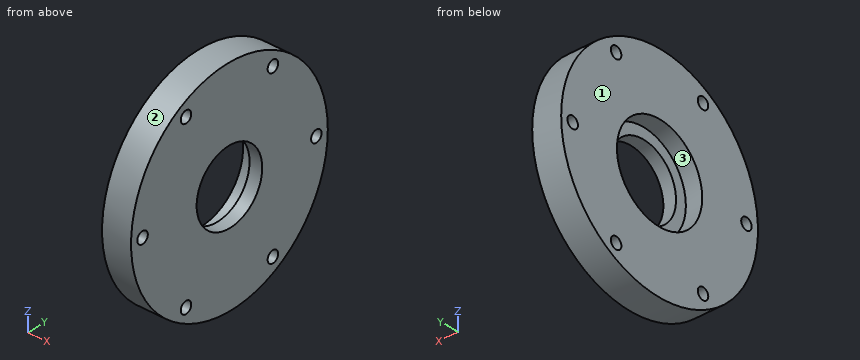
Solid Edge part; units mm, degrees
sketch "Sketch1" plane through (0, 0, 0) normal (1, 0, 0) x (0, 1, 0)
  circle A0 centre (0, 0) radius 10
  circle A1 centre (0, 0) radius 30
extrude "Protrusion1" add sketch "Sketch1" along normal blind 8
sketch "Sketch2" plane through (0, 0, 0) normal (-1, 0, 0) x (0, -1, 0)
  circle A0 centre (0, 0) radius 13
extrude "ExtrudedCutout_1" cut sketch "Sketch2" against normal blind 4.5
sketch "Sketch3" plane through (8, 0, 0) normal (1, 0, 0) x (0, 1, 0)
  circle A0 centre (-26.5, 0) radius 1.6
extrude "Cutout1" cut sketch "Sketch3" against normal up to next
pattern_circular "Pattern1" count 6 over 360 about axis through (8, 0, 0) along (-1, 0, 0) of "Cutout1"
CAD build for the part. Positions are in the model's coordinates, mm. Face numbers are marked on the shaded views. Round coordinates to 2 decimals unless told otherwise and drop trailing zeros. Loops run counter-clockwise (first coordinate to the right, second up) from the corner with the lowest first, then second, coordinate; pieces in that order, holes last.
(1) Wall check: line 1 along Z through (x, y) = (1, 0); line 2 along Z through (x, y) = (5.6, 0); line 3 along Y through (x, z) = (6, 24). Give the ranges that are in metal, low to high.
(2) Cut at C-C (y = -8). Give the cut face in (x, z), plus the area to 3 significant figures.
(3) Cut at A-A (y = 0). Give the cut face in (x, z).
(4) Cut at B-B (x = 5.25). Give the cut face in (y, z).
(5) Drop flat-ended pins along their axis: pin 1 (1.5 mm diameter, centred on x = 4, z = 5.5, fed in from +Y); pin 2 (2.5 mm diameter, centred on y = 26.5, z = 0, fed in from +X); pin 3 (23.5 mm diameter, centred on y = 0, z = 0, fed in from -X); pin 4 (1.5 mm diameter, centred on x = 7, z = 16.5, fed in from +Y). Give the stop position or say it passes through.
(6) Two-plate mould, pull along Y, no slides. Class the marked faces 1, 2 and 3: +Y half, -Y half, draft (parallel to the pull), parting line (faces both ways), or undercut.
(7) Cut at D-D (z = -17.5). Give the cut face in (x, y), plus the area to 3 significant figures.
Findings below:
1. line 1: z = -30 to -13, 13 to 30
1. line 2: z = -30 to -10, 10 to 30
1. line 3: y = -18 to -14.46, -12.04 to 12.04, 14.46 to 18
2. outline: (0, -28.91) - (8, -28.91) - (8, -6) - (4.5, -6) - (4.5, -10.25) - (0, -10.25) - close; (0, 10.25) - (4.5, 10.25) - (4.5, 6) - (8, 6) - (8, 28.91) - (0, 28.91) - close
2. area: 328 mm2
3. outline: (0, -30) - (8, -30) - (8, -10) - (4.5, -10) - (4.5, -13) - (0, -13) - close; (0, 13) - (4.5, 13) - (4.5, 10) - (8, 10) - (8, 30) - (0, 30) - close
4. outline: circle Ø60 at (0, 0); hole circle Ø3.2 at (-26.5, 0); hole circle Ø3.2 at (-13.25, -22.95); hole circle Ø3.2 at (-13.25, 22.95); hole circle Ø20 at (0, 0); hole circle Ø3.2 at (13.25, -22.95); hole circle Ø3.2 at (13.25, 22.95); hole circle Ø3.2 at (26.5, 0)
5. pin 1: stops at y = 29.62
5. pin 2: passes through
5. pin 3: stops at x = 4.5
5. pin 4: stops at y = 25.53
6. face 1: draft
6. face 2: parting line
6. face 3: undercut
7. outline: (0, -24.37) - (8, -24.37) - (8, 24.37) - (0, 24.37) - close
7. area: 390 mm2
